For this review, take the finished solid that the model builds, in its own axes (mm). Face numbers are marked on the shaded views. A direction names the side the tool comes from. Give positions to 0.01 mm unless a question says otherwise; leave off trailing zeros. Order: outer loops, then holes, each group sorted by start corner. A loop starts at its lowest first (then second) coordinate and runs counter-clockwise, first axis right, second up. Notation, with made-up numbers: (-20, -33) - (8, -33) arc R19 cw to (8, -17) - close; hole circle Ø6 at (32.5, -12). An arc over 180 degrees is marked (long way). Put each result on its own line as item: value. Start each with the question number.
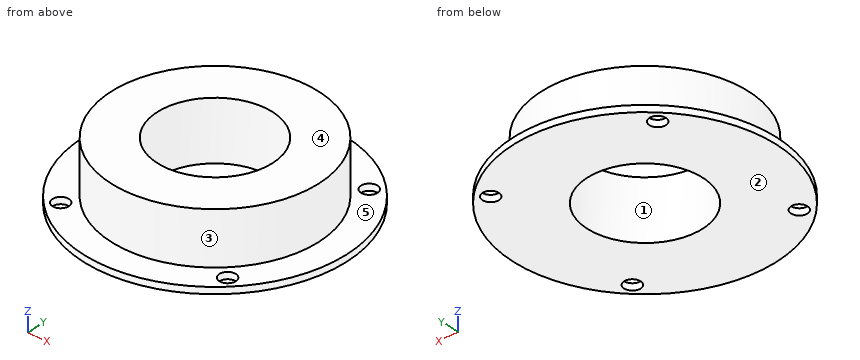
```python
from build123d import *

# Parameters (mm, degrees)
SKETCH2_R           = 40
SKETCH2_R_2         = 17.5
BOSS_EXTRUDE1_DEPTH = 2
SKETCH3_R           = 31.5
SKETCH3_R_2         = 17.5
BOSS_EXTRUDE2_DEPTH = 16
SKETCH5_R           = 2.5
CUT_EXTRUDE1_DEPTH  = 59.787753827


with BuildPart() as part:
    # Sketch2 → Boss-Extrude1 (new body)
    with BuildSketch(Plane.XY):
        Circle(SKETCH2_R)
        Circle(SKETCH2_R_2, mode=Mode.SUBTRACT)
    extrude(amount=BOSS_EXTRUDE1_DEPTH)

    # Sketch3 → Boss-Extrude2 (add)
    with BuildSketch(Plane.XY.offset(2)):
        Circle(SKETCH3_R)
        Circle(SKETCH3_R_2, mode=Mode.SUBTRACT)
    extrude(amount=BOSS_EXTRUDE2_DEPTH)

    # Sketch5 → Cut-Extrude1 (cut, through all)
    with BuildSketch(Plane.XY.offset(2)):
        with Locations((25.455844123, 25.455844123)):
            Circle(SKETCH5_R)
        with Locations((25.455844123, -25.455844123)):
            Circle(SKETCH5_R)
        with Locations((-25.455844123, -25.455844123)):
            Circle(SKETCH5_R)
        with Locations((-25.455844123, 25.455844123)):
            Circle(SKETCH5_R)
    extrude(amount=-CUT_EXTRUDE1_DEPTH, mode=Mode.SUBTRACT)


solid = part.part
```
1. The part is to be moulded in two halves that separate along Y. For the marked faces 1, 2 and 3, say which applies: released by +Y, released by -Y, zero draft, split by the parting line, or undercut.
2. Add section C-C, the plane z = 16.25. Give the boundary of the cut face in (x, y).
3. Add section A-A, the plane y = 0. Give the boundary of the cut face in (x, z).
4. Wall thickness on line 1 (X direction, y = -0.5, z = 4); line 2 (Y direction, x = 0, z = 7); line 3 (Y direction, x = 13, z = 10.5): over which ranges is each line inside the solid? List them lowest first. Write a range as from..to.
5. Tool access review of the marked faces 4 and 5: name each direction out of +Z, -Z, +X, -X, +Y, -Y from which nothing blocks a thin tool from reaching the whole face with its end or side.
6. Clearance check with flat-ended pins moving along their axes: pin 1 (4 mm diameter, centred on x = 28.5, z = 8, fed in from -Y); pin 2 (1.5 mm diameter, centred on y = -13.5, z = 7.5, fed in from -X); pin 3 (8 mm diameter, centred on y = -29.5, z = 15, fed in from -X); pin 4 (4.5 mm diameter, centred on x = 25.46, y = -25.46, fed in from -Z). State where each tip first meets the part, or that it passes through.
7. Add section D-D, the plane x = 29.5. Give the boundary of the cut face in (y, z).
Found:
1. face 1: undercut
1. face 2: zero draft
1. face 3: split by the parting line
2. outline: circle Ø63 at (0, 0); hole circle Ø35 at (0, 0)
3. outline: (-40, 0) - (-17.5, 0) - (-17.5, 18) - (-31.5, 18) - (-31.5, 2) - (-40, 2) - close; (17.5, 0) - (40, 0) - (40, 2) - (31.5, 2) - (31.5, 18) - (17.5, 18) - close
4. line 1: x = -31.5..-17.49, 17.49..31.5
4. line 2: y = -31.5..-17.5, 17.5..31.5
4. line 3: y = -28.69..-11.72, 11.72..28.69
5. face 4: +Z, +X, -X, +Y, -Y
5. face 5: +Z
6. pin 1: stops at y = -17.03
6. pin 2: stops at x = -28.8
6. pin 3: stops at x = -18.49
6. pin 4: passes through
7. outline: (-27.01, 0) - (27.01, 0) - (27.01, 2) - (11.05, 2) - (11.05, 18) - (-11.05, 18) - (-11.05, 2) - (-27.01, 2) - close
